Can you work these out from the model? Positions are in its coordinate system, mm. Round coordinates to 2 decimals unless told otherwise and drop trailing zeros. Loops run counter-clockwise (first coordinate to the right, second up) from the corner with the lowest first, then second, coordinate; pieces in that order, holes last. Notation, with made-up numbers: (80.5, -21.5) -> (93.5, -21.5) arc R34 cw to (93.5, 13.5) -> close; hole circle Ø3 at (14.5, -14). An arc over 180 degrees is marked (long way). Answer as a JSON object with one key per item and string values.
```python
from build123d import *

# Parameters (mm, degrees)
SKETCH1_W           = 28
SKETCH1_H           = 20
BOSS_EXTRUDE1_DEPTH = 3
M3_TAPPED_HOLE1_D   = 2.5


with BuildPart() as part:
    # Sketch1 → Boss-Extrude1 (new body)
    with BuildSketch(Plane(origin=(0, 0, 0), x_dir=(1, 0, 0), z_dir=(0, 1, 0))):
        Rectangle(SKETCH1_W, SKETCH1_H)
    extrude(amount=BOSS_EXTRUDE1_DEPTH)

    # M3 Tapped Hole1 (through all)
    with Locations(Plane(origin=(0, 0, 0), x_dir=(-1, 0, 0), z_dir=(0, -1, 0))):
        with Locations((-11, 7), (10, 7), (10, -7), (-11, -7)):
            Hole(M3_TAPPED_HOLE1_D / 2)


solid = part.part
```
Q1. I want a section at A-A, the plane z = 7. Write out the boundary of the cut face in (x, y), then the cut area to 3 significant figures.
Determined:
{"outline": "(-14, 0) -> (-11.25, 0) -> (-11.25, 3) -> (-14, 3) -> close; (-8.75, 0) -> (9.75, 0) -> (9.75, 3) -> (-8.75, 3) -> close; (12.25, 0) -> (14, 0) -> (14, 3) -> (12.25, 3) -> close", "area": "69.0 mm²"}
Q2. If I drill on L1, parallel to X at y = 2.05, z = -7; L2, parallel to Z at x = 11, y = 0.7; L3, parallel to Z at x = 12, y = 2.6, over which ranges is the centre line in solid material (lowest first)? Write a range as [from, to].
Determined:
{"L1": "[-14, -11.25], [-8.75, 9.75], [12.25, 14]", "L2": "[-10, -8.25], [-5.75, 5.75], [8.25, 10]", "L3": "[-10, -7.75], [-6.25, 6.25], [7.75, 10]"}
Q3. We'd pull the mould along Z, two halves only. Please class faces 1 (the flat face through (0, 1, -10)), 2 (the flat face through (14, 1, 0)), 3 (the cylindrical face through (-11.25, 1.52, 6.95)): pulls with the +Z half, pulls with the -Z half, needs draft (parallel to the pull), parting line crosses it, or undercut.
Determined:
{"face 1": "pulls with the -Z half", "face 2": "needs draft", "face 3": "undercut"}
Q4. I want a section at B-B, the plane x = -10. Write out the boundary of the cut face in (y, z).
Determined:
{"outline": "(0, -10) -> (3, -10) -> (3, -8.25) -> (0, -8.25) -> close; (0, -5.75) -> (3, -5.75) -> (3, 5.75) -> (0, 5.75) -> close; (0, 8.25) -> (3, 8.25) -> (3, 10) -> (0, 10) -> close"}
Q5. I'm going to push a flat-ended pin straight in: pin 1 (2 mm diameter, centred on x = 11, z = 7, fed in from +Y). Where does the tip first touch, or does it pass through?
Determined:
{"pin 1": "through"}
Q6. I want a section at C-C, the plane y = 1.95. Write out the boundary of the cut face in (x, z), then the cut area to 3 significant figures.
Determined:
{"outline": "(-14, -10) -> (14, -10) -> (14, 10) -> (-14, 10) -> close; hole circle Ø2.5 at (-10, -7); hole circle Ø2.5 at (-10, 7); hole circle Ø2.5 at (11, -7); hole circle Ø2.5 at (11, 7)", "area": "540 mm²"}
